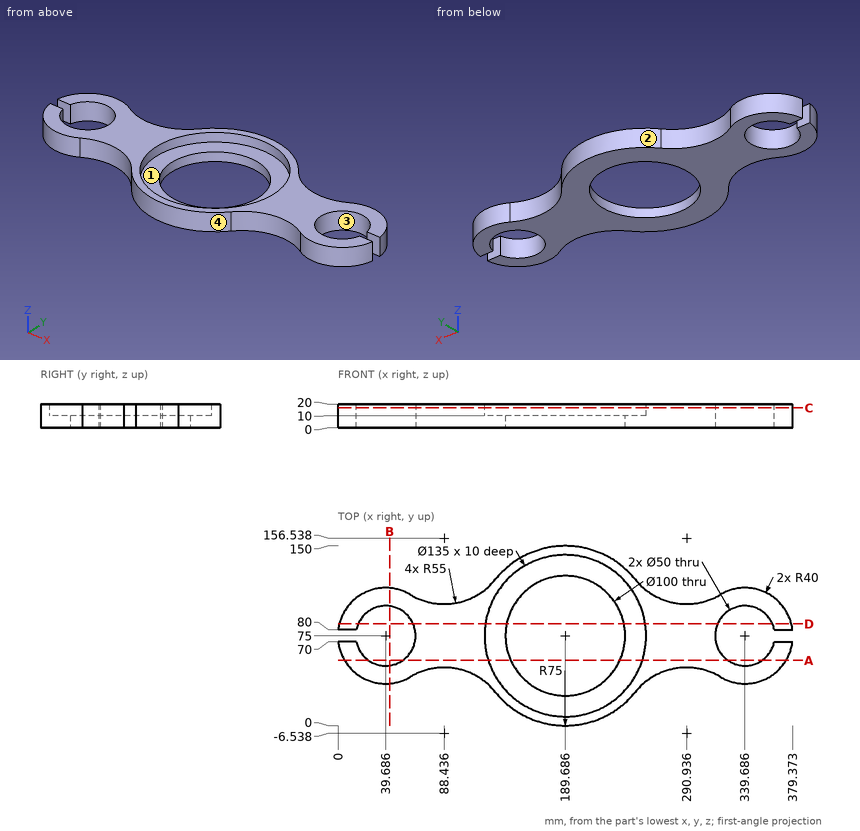
Design review of the part shown in the three views and the two pictorial views. Dimensions are in mm from the part's minimum x, y and z. Give positions to 0.01 mm unless a question says otherwise; leave off trailing zeros. Loops run counter-clockwise (first coordinate to the right, second up) from the corner with the lowest first, then second, coordinate; pieces in that order, holes last. Notation, with made-up numbers: M 10.5,-20.75 L 66.5,-20.75 A18 cw 66.5,10.25 Z; hole C 69,28 d7. An arc over 180 degrees is marked long. Answer as a JSON object with one key per item and string values. Group by question number.
Q1. Add section B-B on x = 43. Give the boundary of the cut face in (y, z), and give its area (3 significant figures).
Q2. Mouldability with a two-part tool opening along Y and no side actions: class the marked faces 1, 2, 3 and 4 as +Y half, -Y half, draft (parallel to the pull), parting line (faces both ways), or undercut.
Q3. Add section A-A on y = 54.5. Give the boundary of the cut face in (x, z) (1 decimal).
Q4. Add section C-C on z = 16.75. Give the boundary of the cut face in (x, y), and give its area (3 significant figures).
Q5. For probe 1 along X at (y, z) = (69, 3.25) (1 decimal); probe 2 along X at (y, z) = (95, 9.5) (1 decimal); probe 3 along Z at (x, y) = (169, 129), list the stretches that pass through material, from the lowest coordinate up. Write a range as [from, to].
Q6. Add section D-D on y = 85. Give the boundary of the cut face in (x, z), and give its area (3 significant figures).
Q7. Insertion check: P1, Ø8, axis at y = 97.5, z = 10, coming from the +X side; P2, Ø4, axis at y = 110.5, z = 4.5, coming from the -X side; P3, Ø12, axis at x = 371, z = 9, coming from the +Y side. Each pin has a flat end and moves straight along its axis. Give the tip position at first contact, or say it passes through.
Checked values:
{
 "1": {"outline": "M 35.14,0 L 50.22,0 L 50.22,20 L 35.14,20 Z; M 99.78,0 L 114.86,0 L 114.86,20 L 99.78,20 Z", "area": "603 mm²"},
 "2": {"face 1": "undercut", "face 2": "+Y half", "face 3": "undercut", "face 4": "-Y half"},
 "3": {"outline": "M 5.3,0 L 25.4,0 L 25.4,20 L 5.3,20 Z; M 54,0 L 144.1,0 L 144.1,10 L 125.4,10 L 125.4,20 L 54,20 Z; M 235.3,0 L 325.4,0 L 325.4,20 L 254,20 L 254,10 L 235.3,10 Z; M 354,0 L 374,0 L 374,20 L 354,20 Z"},
 "4": {"outline": "M 0,70 A40 ccw 60.21,40.67 A55 cw 131.27,27.96 A75 ccw 248.1,27.96 A55 cw 319.16,40.67 A40 ccw 379.37,70 L 364.18,70 A25 cw long 364.18,80 L 379.37,80 A40 ccw 319.16,109.33 A55 cw 248.1,122.04 A75 ccw 131.27,122.04 A55 cw 60.21,109.33 A40 ccw 0,80 L 15.19,80 A25 cw long 15.19,70 Z; hole C 189.69,75 d135", "area": "14,100 mm²"},
 "5": {"probe 1": "[0.1, 15.4], [64, 140], [239.3, 315.4], [364, 379.2]", "probe 2": "[5, 24.7], [54.7, 143.9], [235.5, 324.7], [354.7, 374.3]", "probe 3": "[0, 10]"},
 "6": {"outline": "M 0.96,0 L 16.77,0 L 16.77,20 L 0.96,20 Z; M 62.6,0 L 140.7,0 L 140.7,10 L 122.93,10 L 122.93,20 L 62.6,20 Z; M 238.68,0 L 316.77,0 L 316.77,20 L 256.44,20 L 256.44,10 L 238.68,10 Z; M 362.6,0 L 378.42,0 L 378.42,20 L 362.6,20 Z", "area": "3,400 mm²"},
 "7": {"P1": "x = 375.15", "P2": "x = 17.83", "P3": "y = 105.97"}
}
